from build123d import *

# Parameters (mm, degrees)
F2_DEPTH = 13.462


with BuildPart() as f2:
    # F0 (on Front) → F2 (new body)
    with BuildSketch(Plane.XZ):
        with BuildLine():
            Line((-42.96492, -18.441067), (-42.96492, -30.318613))
            Line((-42.96492, -30.318613), (58.63508, -30.318613))
            Line((58.63508, -30.318613), (58.63508, 20.481387))
            Line((58.63508, 20.481387), (-42.96492, 20.481387))
            Line((-42.96492, 20.481387), (-42.96492, 8.603842))
            ThreePointArc((-42.96492, 8.603842), (-33.403101, 4.643207), (-29.442466, -4.918613))
            ThreePointArc((-29.442466, -4.918613), (-33.403101, -14.480432), (-42.96492, -18.441067))
        make_face()
        with BuildLine():
            ThreePointArc((-42.96492, 20.481387), (-68.36492, -4.918613), (-42.96492, -30.318613))
            Line((-42.96492, -30.318613), (-42.96492, -18.441067))
            ThreePointArc((-42.96492, -18.441067), (-56.487375, -4.918613), (-42.96492, 8.603842))
            Line((-42.96492, 8.603842), (-42.96492, 20.481387))
        make_face()
    extrude(amount=F2_DEPTH)


solid = f2.part
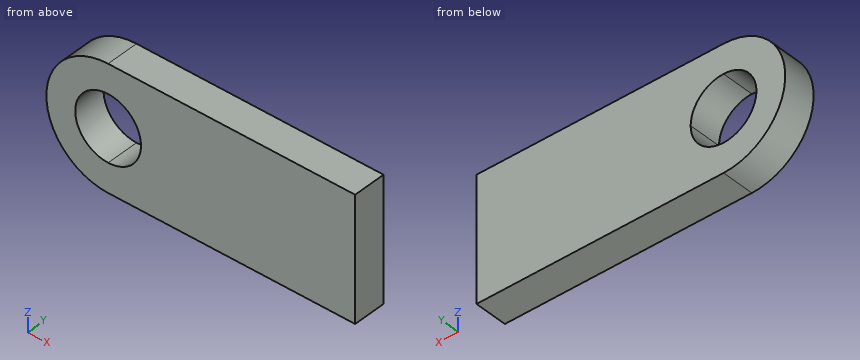
Source: CAD feature listing. Evaluate the final solid. Frame: model axes, mm. Coordinates: 2 decimals unless noted, no trailing zeros. Loops run counter-clockwise (first coordinate to the right, second up) from the corner with the lowest first, then second, coordinate; pieces in that order, holes last. Notation, with made-up numbers: M 58,-6 L 103,-6 A29 ccw 103,28 Z; hole C 77.5,82.25 d11. An arc over 180 degrees is marked long. Answer in a Markdown table with one row per item.
Q1. Ray query, probe 1 along X at (y, z) = (-9.5, 2.5); probe 2 along Z at (x, y) = (-46, -11.25); probe 3 along X at (y, z) = (-1.75, -12.5). Return the intervals inside material, ascending. Write a range as from..to.
Answers below:
| item | result |
|---|---|
| probe 1 | x = -67.26..-54.27, -31.66..58.64 |
| probe 2 | z = -30.14..-18.1, 8.26..20.3 |
| probe 3 | x = -67.21..-54.16, -31.77..58.64 |
Q2. Section D-D on x = -58.5. Return the cut outline in (y, z).
Answers below:
| item | result |
|---|---|
| outline | M -13.46,-25.01 L 0,-25.01 L 0,15.18 L -13.46,15.18 Z |
Q3. Section C-C on z = -17. Return the cut outline in (x, y).
Answers below:
| item | result |
|---|---|
| outline | M -65.31,-13.46 L -49.04,-13.46 L -49.04,0 L -65.31,0 Z; M -36.89,-13.46 L 58.64,-13.46 L 58.64,0 L -36.89,0 Z |
Q4. Section B-B on y = -4.25. Return the cut outline in (x, z), plus the area to 3 significant figures.
Answers below:
| item | result |
|---|---|
| outline | M -42.96,-30.32 L 58.64,-30.32 L 58.64,20.48 L -42.96,20.48 A25.4 ccw Z; hole M -42.96,-18.44 A13.52 ccw -29.44,-4.92 A13.52 ccw long Z |
| area | 5,600 mm^2 |
Q5. First-contact query: pin 1 (5 mm diameter, centred on y = -8.5, z = -10.5, fed in from -X); pin 2 (4 mm diameter, centred on y = -3.5, z = 3, fed in from -X). Flat tips, straight axial feed; report the tip coordinate or a pass-through.
Answers below:
| item | result |
|---|---|
| pin 1 | stops at x = -68.18 |
| pin 2 | stops at x = -67.67 |
Q6. Section A-A on z = -3. Return the cut outline in (x, y), plus the area to 3 significant figures.
Answers below:
| item | result |
|---|---|
| outline | M -68.29,-13.46 L -56.35,-13.46 L -56.35,0 L -68.29,0 Z; M -29.58,-13.46 L 58.64,-13.46 L 58.64,0 L -29.58,0 Z |
| area | 1,350 mm^2 |
